Model file for the job. Use its own axes, mm. A direction names the side the tool comes from. Coordinates: 2 decimals unless noted, no trailing zeros. Write each loop counter-clockwise with the first axis right and the second up, starting at its lowest first coordinate (ties: lowest second). Pieces come first, ordered by that corner, then holes. Notation, with made-up numbers: (19.5, 12.5) -> (57.5, 12.5) arc R6 ccw to (57.5, 17.5) -> close; hole circle Ø3 at (61, 23). An arc over 180 degrees is marked (long way). Answer as a JSON object with one key per item and string values. Group by question number.
Autodesk Fusion 360 part; units mm, degrees
sketch "Sketch1" plane through (0, 0, 0) normal (0, 1, 0) x (1, 0, 0)
  line L0 (0, 0) -> (40, 0)
  line L1 (40, 0) -> (40, -8)
  line L2 (40, -8) -> (0, -8)
  line L3 (0, -8) -> (0, 0)
  line L4 (0, 0) -> (14.3059, 42.6654)
  line L5 (14.3059, 42.6654) -> (21.8909, 40.1222)
  line L6 (21.8909, 40.1222) -> (8.4377, 0)
  dimension "d1" = 40
  dimension "d2" = 8
  dimension "d4" = 8
  dimension "d5" = 71.463
  dimension "d9" = 45
extrude "Extrude3" add sketch "Sketch1" along normal blind 3
fillet "Fillet8" radius 3 4 edges at (0, 1.5, 8) (0, 1.5, 0) (14.3059, 1.5, -42.6654) (21.8909, 1.5, -40.1222)
sketch "Sketch4" plane through (0, 0, 0) normal (0, -1, 0) x (1, 0, 0)
  arc A0 (19.0465, -41.0759) -> (20.9372, -37.2778) centre (18.0928, -38.2315) ccw
  line L0 (20.9372, -37.2778) -> (8.4377, 0)
  line L1 (8.4377, 0) -> (40, 0)
  line L2 (40, 0) -> (40, 8)
  line L3 (40, 8) -> (3, 8)
  arc A1 (3, 8) -> (0, 5) centre (3, 5) ccw
  line L4 (0, 5) -> (0, 0.4896)
  arc A2 (0, 0.4896) -> (0.1556, -0.4642) centre (3, 0.4896) ccw
  line L5 (0.1556, -0.4642) -> (13.3522, -39.8211)
  arc A3 (13.3522, -39.8211) -> (17.1503, -41.7117) centre (16.1966, -38.8674) ccw
  line L6 (17.1503, -41.7117) -> (19.0465, -41.0759)
  line L7 (40, 8) -> (30, 8)
  line L8 (30, 8) -> (30, 0)
  line L9 (30, 0) -> (40, 0)
  line L10 (40, 0) -> (40, 8)
  dimension "d26" = 10
extrude "Extrude4" add sketch "Sketch4" along normal blind 3 and the other way blind 6 contours L1 L2 L3 L7 L8 L9 L10
fillet "Fillet9" radius 6 1 edges at (40, 1.5, 8)
fillet "Fillet10" radius 1 1 edges at (40, 1.5, 0)
fillet "Fillet11" radius 1 2 edges at (30, 0, 4) (30, 3, 4)
extrude "Extrude1" [suppressed]
moveface "MoveFace1" [suppressed]
fillet "Fillet1" [suppressed]
fillet "Fillet2" [suppressed]
sketch "Sketch2" plane through (0, 0, 0) normal (0, 1, 0) x (1, 0, 0)
  line L0 (40, -8) -> (31, -8)
  line L1 (31, -8) -> (31, 0)
  line L2 (31, 0) -> (40, 0)
  line L3 (40, 0) -> (40, -8)
  line L4 (40, 0) -> (40, -8)
  dimension "d12" = 9
  dimension "d13" = 8
extrude "Extrude2" [suppressed]
fillet "Fillet3" [suppressed]
fillet "Fillet4" [suppressed]
fillet "Fillet5" [suppressed]
sketch "Sketch3" plane through (0, 0, 0) normal (0, 1, 0) x (1, 0, 0)
delete_face "DeleteFace1" [suppressed]
fillet "Fillet6" [suppressed]
delete_face "DeleteFace2" [suppressed]
fillet "Fillet7" [suppressed]
(1) Pin check, flat tips, straight feed: pin 1 (1 mm diameter, centred on y = -2.5, z = 4, fed in from -X); pin 2 (10 mm diameter, centred on x = 5, z = -13, fed in from +Y); pin 3 (12 mm diameter, centred on x = 10, z = -21, fed in from -Y); pin 4 (12 mm diameter, centred on x = 22.5, z = -10.5, fed in from -Y). Stop position of each tip, or through.
(2) Cut at B-B on y = 0.75. List the corners of the cut face in (x, z), plus the area to 3 significant figures.
(3) Wall check: probe 1 along Y at (x, z) = (11.5, -32.5); probe 2 along X at (y, z) = (4.75, 1); probe 3 along Z at (x, y) = (21.5, 2.75). Give the ranges that are in metal, low to high.
(4) Cut at A-A on x = 18.5. List the corners of the cut face in (y, z).
(5) 3-axis set-ups, long thin cutter, end or side, ignore diameter. For faces 5 (the face through (30, 5, 4)), 6 (the face through (27, 1, 0)), 7 (the face through (14.89, 1.52, -41.57)): which of +Z, -Z, +X, -X, +Y, -Y reach the whole face in a straight line?
(6) Cut at D-D on z = -8. List the corners of the cut face in (x, y).
(7) Cut at C-C on x = 25.5. List the corners of the cut face in (y, z).
(8) Pull direction Z, two halves, no side cores. Call faces 1 (the face through (22, 1, 8)), 2 (the face through (14.775, 1.479, -18.9)), 3 (the face through (20.793, 1.521, -39.539)), 4 (the face through (18.085, 1.479, -41.398)): released by +Z, released by -Z, zero draft, split by the parting line, or undercut.
Results found:
{
 "1": {"pin 1": "stops at x = 30", "pin 2": "stops at y = 3", "pin 3": "stops at y = 0", "pin 4": "passes through"},
 "2": {"outline": "(0, 0.49) arc R3 ccw to (0.16, -0.46) -> (13.35, -39.82) arc R3 ccw to (17.15, -41.71) -> (19.05, -41.08) arc R3 ccw to (20.94, -37.28) -> (8.44, 0) -> (39, 0) arc R1 ccw to (40, 1) -> (40, 2) arc R6 ccw to (34, 8) -> (3, 8) arc R3 ccw to (0, 5) -> close", "area": "656 mm²"},
 "3": {"probe 1": "y = 0 to 3", "probe 2": "x = 30 to 40", "probe 3": "z = 0 to 8"},
 "4": {"outline": "(0, -41.26) -> (3, -41.26) -> (3, -30.01) -> (0, -30.01) -> close; (0, 0) -> (3, 0) -> (3, 8) -> (0, 8) -> close"},
 "5": {"face 5": "+Z, -Z, -X, +Y", "face 6": "+X, +Y, -Y", "face 7": "-Z, +Y, -Y"},
 "6": {"outline": "(2.68, 0) -> (11.12, 0) -> (11.12, 3) -> (2.68, 3) -> close"},
 "7": {"outline": "(0, 0) -> (3, 0) -> (3, 8) -> (0, 8) -> close"},
 "8": {"face 1": "released by +Z", "face 2": "undercut", "face 3": "undercut", "face 4": "released by -Z"}
}
